Geometry: final body of the model. Coordinates: model frame, mm. Face numbers are marked on the shaded views. Give positions to 0.01 mm unless a question says otherwise; leave off trailing zeros. Order: outer loops, then holes, each group sorted by start corner. A loop starts at its lowest first (then second) coordinate and runs counter-clockwise, first axis right, second up. Notation, with made-up numbers: (-13.75, 38.5) - (-7.75, 38.5) arc R22 cw to (-7.75, 59.5) - close; hole circle Ø2 at (53, 9). An arc over 180 degrees is marked (long way). Use one line per item in the form item = value.
from build123d import *

# Parameters (mm, degrees)
F0_R     = 0.75
F1_DEPTH = 1


with BuildPart() as f1:
    # F0 (on Top) → F1 (new body)
    with BuildSketch(Plane.XY):
        with BuildLine():
            Line((-8.068125, -4.2), (-9.313614, -4.84836))
            ThreePointArc((-9.313614, -4.84836), (0, -10.5), (9.313614, -4.84836))
            Line((9.313614, -4.84836), (8.068125, -4.2))
            Line((8.068125, -4.2), (5.848077, -4.2))
            ThreePointArc((5.848077, -4.2), (0, -7.2), (-5.848077, -4.2))
            Line((-5.848077, -4.2), (-8.068125, -4.2))
        make_face()
        with Locations((0, -8.2)):
            Circle(F0_R, mode=Mode.SUBTRACT)
        with Locations((-5.3, -6.256996)):
            Circle(F0_R, mode=Mode.SUBTRACT)
        with Locations((5.3, -6.256996)):
            Circle(F0_R, mode=Mode.SUBTRACT)
    extrude(amount=F1_DEPTH)


solid = f1.part
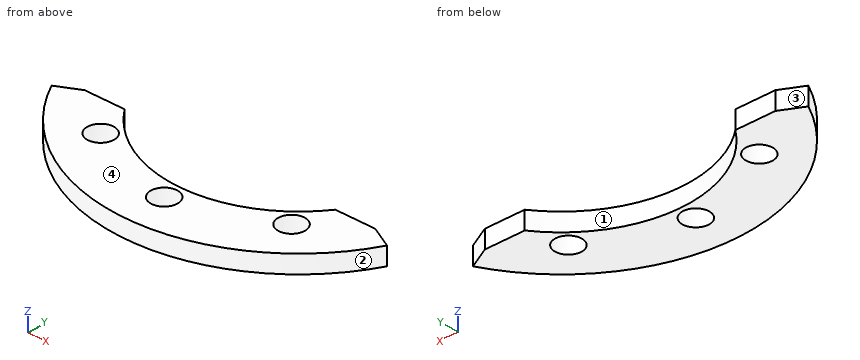
(1) Ray query, line 1 along Y through (x, z) = (5.3, 0.5); line 2 along X through (y, z) = (-4.5, 0.1); line 3 along X through (y, z) = (-4.75, 0.9). Return the intervals inside material, ascending.
Computed values:
line_1 = -9.06 to -7.01, -5.51 to -4.87
line_2 = -8.64 to -5.62, 5.62 to 8.64
line_3 = -9.12 to -5.41, 5.41 to 9.12
(2) Cut plane B-B on y = -5.75. Output: boundary loops of the cut face in (x, z).
Computed values:
outline = (-8.79, 0) - (-5.85, 0) - (-5.85, 1) - (-8.79, 1) - close; (-4.75, 0) - (-4.33, 0) - (-4.33, 1) - (-4.75, 1) - close; (4.33, 0) - (4.75, 0) - (4.75, 1) - (4.33, 1) - close; (5.85, 0) - (8.79, 0) - (8.79, 1) - (5.85, 1) - close
(3) Cut plane D-D on y = -8.2. Output: boundary loops of the cut face in (x, z), plus the area to 3 significant figures.
Computed values:
outline = (-6.56, 0) - (-0.75, 0) - (-0.75, 1) - (-6.56, 1) - close; (0.75, 0) - (6.56, 0) - (6.56, 1) - (0.75, 1) - close
area = 11.6 mm²
(4) Cut plane A-A on x = 0. Output: boundary loops of the cut face in (y, z).
Computed values:
outline = (-10.5, 0) - (-8.95, 0) - (-8.95, 1) - (-10.5, 1) - close; (-7.45, 0) - (-7.2, 0) - (-7.2, 1) - (-7.45, 1) - close
(5) Pull-direction query (X, two-part tool) for the marked faces 1, 2, 3 and 4; classes: released by +X, released by -X, zero draft, split by the parting line, or undercut.
Computed values:
face_1 = undercut
face_2 = split by the parting line
face_3 = released by -X
face_4 = zero draft
(6) Cut plane C-C on z = 0.55. Output: boundary loops of the cut face in (x, y).
Computed values:
outline = (-9.31, -4.85) arc R10.5 ccw to (9.31, -4.85) - (8.07, -4.2) - (5.85, -4.2) arc R7.2 cw to (-5.85, -4.2) - (-8.07, -4.2) - close; hole circle Ø1.5 at (-5.3, -6.26); hole circle Ø1.5 at (0, -8.2); hole circle Ø1.5 at (5.3, -6.26)
